from build123d import *

# Parameters (mm, degrees)
BOSS_EXTRU_1_DEPTH           = 450
CHANFREIN1_SIZE              = 0.25
CHANFREIN1_OF_SYM_TRIE1_SIZE = 0.25
ESQUISSE2_R                  = 3
ENL_V_MAT_EXTRU_1_DEPTH      = 4
ESQUISSE3_R                  = 1.65
ENL_V_MAT_EXTRU_2_DEPTH      = 451.057774069
R_P_TITION_LIN_AIRE1_COUNT   = 18
R_P_TITION_LIN_AIRE1_PITCH   = 25


with BuildPart() as part:
    # Esquisse1 → Boss.-Extru.1 (new body)
    with BuildSketch(Plane(origin=(0, 0, 0), x_dir=(0, 0, -1), z_dir=(1, 0, 0))):
        Polygon((6, 5), (6, 0), (0, 0), (0, 8), (6, 8), (6, 6), (4.4, 6), (4.4, 5), align=None)
    boss_extru_1 = extrude(amount=BOSS_EXTRU_1_DEPTH)

    # Chanfrein1
    chanfrein1_edges = [part.edges().sort_by_distance(p)[0] for p in [
        (225, 6, -6),
        (225, 5, -6),
        (225, 0, -6),
        (225, 8, -6),
    ]]
    chamfer(chanfrein1_edges, length=CHANFREIN1_SIZE)

    # Symétrie1: Boss.-Extru.1 across plane
    add(boss_extru_1.mirror(Plane.XY))

    # Chanfrein1 of Symétrie1
    chanfrein1_of_sym_trie1_edges = [part.edges().sort_by_distance(p)[0] for p in [
        (225, 6, 6),
        (225, 5, 6),
        (225, 0, 6),
        (225, 8, 6),
    ]]
    chamfer(chanfrein1_of_sym_trie1_edges, length=CHANFREIN1_OF_SYM_TRIE1_SIZE)

    # Esquisse2 → Enlèv. mat.-Extru.1 (cut)
    with BuildSketch(Plane(origin=(0, 8, 0), x_dir=(1, 0, 0), z_dir=(0, 1, 0))):
        with Locations(Location((11.153483455, 0, 0), (0, 0, 270))):
            Circle(ESQUISSE2_R)
    enl_v_mat_extru_1 = extrude(amount=-ENL_V_MAT_EXTRU_1_DEPTH, mode=Mode.SUBTRACT)

    # Esquisse3 → Enlèv. mat.-Extru.2 (cut, through all)
    with BuildSketch(Plane(origin=(0, 4, 0), x_dir=(1, 0, 0), z_dir=(0, 1, 0))):
        with Locations(Location((11.153483455, 0, 0), (0, 0, 270))):
            Circle(ESQUISSE3_R)
    enl_v_mat_extru_2 = extrude(amount=-ENL_V_MAT_EXTRU_2_DEPTH, mode=Mode.SUBTRACT)

    # Répétition linéaire1: Enlèv. mat.-Extru.1, Enlèv. mat.-Extru.2 ×18
    with Locations(*[(i * R_P_TITION_LIN_AIRE1_PITCH, 0, 0) for i in range(1, R_P_TITION_LIN_AIRE1_COUNT)]):
        add(enl_v_mat_extru_1, mode=Mode.SUBTRACT)
        add(enl_v_mat_extru_2, mode=Mode.SUBTRACT)


solid = part.part
Build history of the part. All positions in model axes, mm. Coordinates: 2 decimals unless noted, no trailing zeros. Write each loop counter-clockwise with the first axis right and the second up, starting at its lowest first coordinate (ties: lowest second). Pieces come first, ordered by that corner, then holes. Notation, with made-up numbers: (36, 87) -> (66, 87) arc R20 cw to (66, 106) -> close; hole circle Ø7 at (49, 47.5). An arc over 180 degrees is marked (long way). Use CSV: the item, a comma, the result in double quotes. Start each with the question number.
Q1. Drill centre lines: probe 1 along Z at (x, y) = (86, 4.25); probe 2 along Y at (x, z) = (74.5, -5.5); probe 3 along Z at (x, y) = (161, 0.5). Where is each one in solid material? Low to high.
Q2. Flat gauge pins, fed straight in: pin 1 Ø6.5 at (x, z) = (260.5, -0.5) entering from +Y; pin 2 Ø0.8 at (x, y) = (159.5, 5.5) entering from -Z; pin 3 Ø5.5 at (x, z) = (236.15, 0) entering from +Y. Where does each tip first touch, or does it go through?
Q3. Cut at A-A, the plane x = 400. List the corners of the cut face in (y, z).
Checked values:
1,probe 1,"z = -6 to -3, 3 to 6"
1,probe 2,"y = 0 to 5, 6 to 8"
1,probe 3,"z = -6 to -1.64, 1.64 to 6"
2,pin 1,"stops at y = 8"
2,pin 2,"stops at z = -4.4"
2,pin 3,"stops at y = 4"
3,outline,"(0, -5.75) -> (0.25, -6) -> (4.75, -6) -> (5, -5.75) -> (5, -4.4) -> (6, -4.4) -> (6, -5.75) -> (6.25, -6) -> (7.75, -6) -> (8, -5.75) -> (8, 5.75) -> (7.75, 6) -> (6.25, 6) -> (6, 5.75) -> (6, 4.4) -> (5, 4.4) -> (5, 5.75) -> (4.75, 6) -> (0.25, 6) -> (0, 5.75) -> close"
